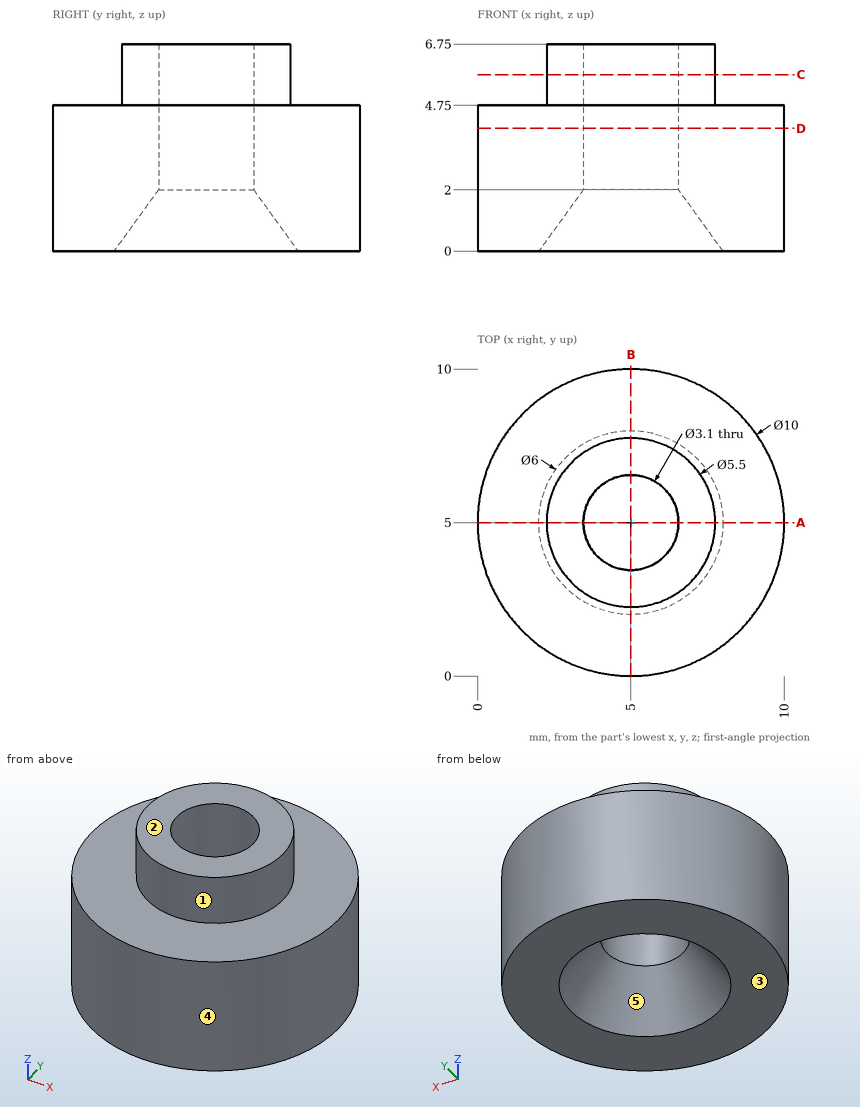
Geometry: see drawing. Coordinates: mm, zero at the bounding-box minimum. A direction names the side the tool comes from. Round coordinates to 2 decimals unless told otherwise and drop trailing zeros. Write each loop counter-clockwise with the first axis right and the second up, starting at its lowest first coordinate (ties: lowest second). Pieces come first, ordered by that corner, then holes.
1) Cut plane A-A (y = 5). Return the cut outline in (x, z), then the cut area to 3 significant figures.
2) Reachability of the marked faces 1 and 2 from +Z, -Z, +X, -X, +Y, -Y: full face, straight path, thin tool, end or side. Return the list, or none.
3) Cut plane D-D (z = 4). Return the cut outline in (x, y).
4) Cut plane C-C (z = 5.75). Return the cut outline in (x, y), then the cut area to 3 significant figures.
5) Ray query, L1, parallel to Y at x = 5, z = 4.4; L2, parallel to Z at x = 5.25, y = 1.5; L3, parallel to Z at x = 7.25, y = 6. Return the intervals inside material, ascending.
6) Contact query for flat-ended pins moving along their axis: P1, Ø1.5, axis at x = 8.5, z = 4.5, coming from the +Y side; P2, Ø1.5, axis at x = 2.5, z = 2, coming from the +Y side; P3, Ø1.5, axis at x = 8, y = 8.5, coming from the +Z side; P4, Ø3, axis at x = 6, y = 1.5, coming from the +Z side. Output: stop coordinate, or through.
7) Draft query along X for the marked faces 3, 4 and 5. Return one class per face: pulls with the +X half, pulls with the -X half, needs draft (parallel to the pull), parting line crosses it, or undercut.
Geometry says:
1. outline: (0, 0) - (2, 0) - (3.45, 2) - (3.45, 6.75) - (2.25, 6.75) - (2.25, 4.75) - (0, 4.75) - close; (6.55, 2) - (8, 0) - (10, 0) - (10, 4.75) - (7.75, 4.75) - (7.75, 6.75) - (6.55, 6.75) - close
1. area: 34.7 mm2
2. face 1: +Z
2. face 2: +Z, +X, -X, +Y, -Y
3. outline: circle Ø10 at (5, 5); hole circle Ø3.1 at (5, 5)
4. outline: circle Ø5.5 at (5, 5); hole circle Ø3.1 at (5, 5)
4. area: 16.2 mm2
5. L1: y = 0 to 3.45, 6.55 to 10
5. L2: z = 0 to 4.75
5. L3: z = 0.74 to 6.75
6. P1: stops at y = 9.18
6. P2: stops at y = 9.68
6. P3: stops at z = 4.75
6. P4: stops at z = 6.75
7. face 3: needs draft
7. face 4: parting line crosses it
7. face 5: undercut
